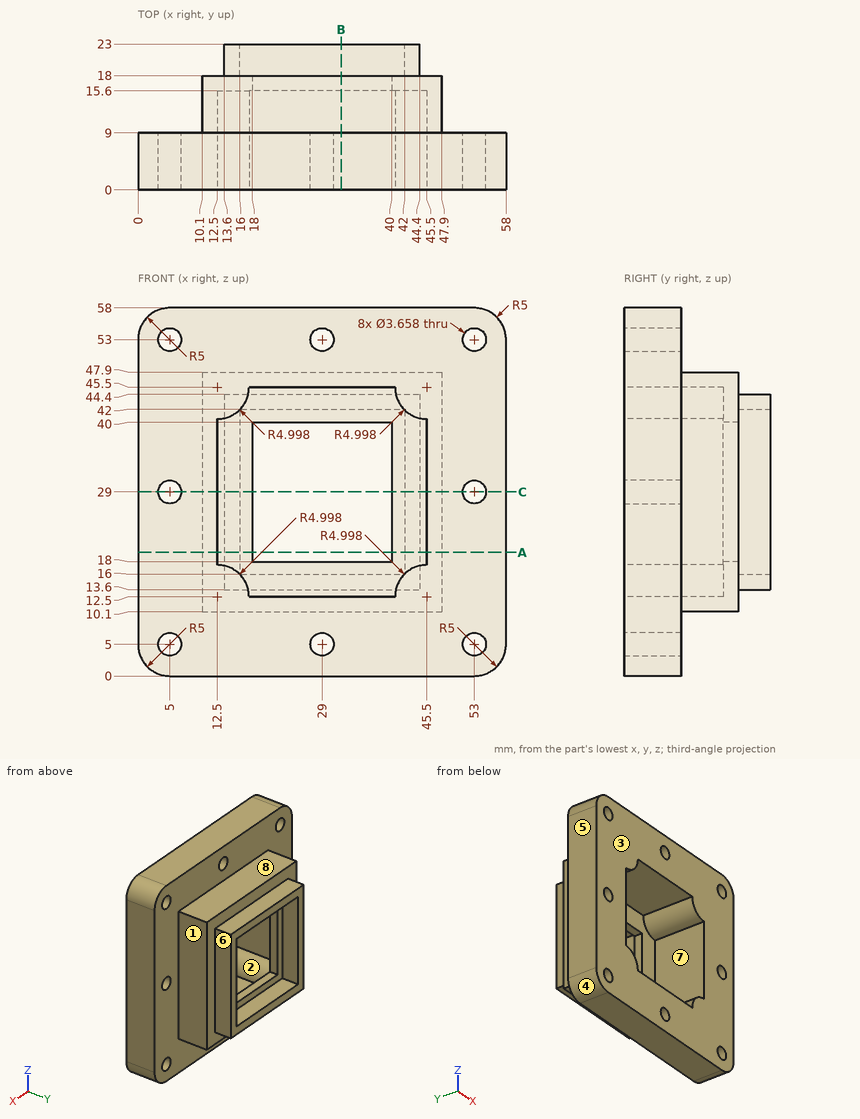
Here's the drawing with two shaded views (mm, measured from the low corner). I have some questions. A direction names the side the tool comes from. Coordinates: 2 decimals unless noted, no trailing zeros. Loops run counter-clockwise (first coordinate to the right, second up) from the corner with the lowest first, then second, coordinate; pieces in that order, holes last. Notation, with made-up numbers: (54.5, 70) -> (105.5, 70) arc R27 ccw to (105.5, 102) -> close; hole circle Ø3 at (-27.75, 25.5). An arc over 180 degrees is marked (long way). Answer as a JSON object with one key per item and string values.
1) For P1, Ø2.5, axis at y = 14, z = 26, coming from the -X side; P2, Ø1.2, axis at x = 27.5, y = 16.5, coming from the -Z side; P3, Ø1.2, axis at y = 17, z = 31, coming from the +X side; P4, Ø1.5, axis at x = 49.5, y = 15.5, coming from the +Z side, each with a flat end and sliding along its axis, tell me the tip position at first contact or that it passes through.
Results:
{"P1": "stops at x = 10.1", "P2": "stops at z = 10.1", "P3": "stops at x = 47.9", "P4": "passes through"}
2) Thinking about a two-plate mould opening in X: for the marked faces 1, 2 and 3, which applies, pulls with the +X half, pulls with the -X half, needs draft (parallel to the pull), parting line crosses it, or undercut?
Results:
{"face 1": "pulls with the +X half", "face 2": "undercut", "face 3": "needs draft"}
3) Imagine slicing it at A-A (z = 19.5). Please give me the cut outline in (x, y).
Results:
{"outline": "(0, 0) -> (12.5, 0) -> (12.5, 15.6) -> (18, 15.6) -> (18, 18) -> (16, 18) -> (16, 23) -> (13.6, 23) -> (13.6, 18) -> (10.1, 18) -> (10.1, 9) -> (0, 9) -> close; (40, 15.6) -> (45.5, 15.6) -> (45.5, 0) -> (58, 0) -> (58, 9) -> (47.9, 9) -> (47.9, 18) -> (44.4, 18) -> (44.4, 23) -> (42, 23) -> (42, 18) -> (40, 18) -> close"}
4) Imagine slicing it at C-C (z = 29). Count the separate pieces of the cut face and the enclosed holes in it, then the cut area to 3 significant figures.
Results:
{"separate pieces": "4", "enclosed holes": "0", "area": "253 mm^2"}
5) If I drill on line 1 (X direction, y = 6, z = 29); line 2 (X direction, y = 2.25, z = 53); line 3 (X direction, y = 20, z = 24.5), over which ranges is the centre line in solid material (lowest first)?
Results:
{"line 1": "x = 0 to 3.17, 6.83 to 12.5, 45.5 to 51.17, 54.83 to 58", "line 2": "x = 0 to 3.17, 6.83 to 27.17, 30.83 to 51.17, 54.83 to 58", "line 3": "x = 13.6 to 16, 42 to 44.4"}
6) For the marked faces 4, 5, 6, 7 and 8, which set-ups out of +Z, -Z, +X, -X, +Y, -Y let a thin tool reach every point of the face, with its end or its side?
Results:
{"face 4": "-Z, -X, +Y, -Y", "face 5": "+Z, -Z, -X, +Y, -Y", "face 6": "+Z, -Z, +X, +Y", "face 7": "-Y", "face 8": "+Z, +X, -X, +Y"}
7) Imagine slicing it at B-B (x = 32). Please give me the cut outline in (y, z).
Results:
{"outline": "(0, 0) -> (9, 0) -> (9, 10.1) -> (18, 10.1) -> (18, 13.6) -> (23, 13.6) -> (23, 16) -> (18, 16) -> (18, 18) -> (15.6, 18) -> (15.6, 12.5) -> (0, 12.5) -> close; (0, 45.5) -> (15.6, 45.5) -> (15.6, 40) -> (18, 40) -> (18, 42) -> (23, 42) -> (23, 44.4) -> (18, 44.4) -> (18, 47.9) -> (9, 47.9) -> (9, 58) -> (0, 58) -> close"}
